Build history of the part. All positions in model axes, mm. Face numbers are marked on the shaded views. A direction names the side the tool comes from. Round coordinates to 2 decimals unless told otherwise and drop trailing zeros. Loops run counter-clockwise (first coordinate to the right, second up) from the corner with the lowest first, then second, coordinate; pieces in that order, holes last. Notation, with made-up numbers: (81.5, 10) - (90.5, 10) arc R24 cw to (90.5, 36) - close; hole circle Ø5 at (-16.5, 8). An arc over 180 degrees is marked (long way). Answer as CSV lines item,"result". Start each with the question number.
```python
from build123d import *

# Parameters (mm, degrees)
SKETCH1_W           = 54.800000096
SKETCH1_H           = 50.990000096
BOSS_EXTRUDE2_DEPTH = 2
SKETCH2_R           = 2
SKETCH2_R_2         = 1
BOSS_EXTRUDE3_DEPTH = 3
SKETCH3_W           = 54.800000096
SKETCH3_H           = 50.990000096
SKETCH3_W_2         = 50.800000096
SKETCH3_H_2         = 46.990000096
BOSS_EXTRUDE5_DEPTH = 47.45


with BuildPart() as part:
    # Sketch1 → Boss-Extrude2 (new body)
    with BuildSketch(Plane(origin=(0, 0, 0), x_dir=(1, 0, 0), z_dir=(0, 1, 0))):
        Rectangle(SKETCH1_W, SKETCH1_H)
    extrude(amount=BOSS_EXTRUDE2_DEPTH)

    # Sketch2 → Boss-Extrude3 (add)
    # profile 1 of 4: a face of its own
    with BuildSketch(Plane(origin=(0, 2, 0), x_dir=(1, 0, 0), z_dir=(0, 1, 0))):
        with Locations(Location((-22.86, 20.955, 0), (0, 0, 90))):
            Circle(SKETCH2_R)
        with Locations(Location((-22.86, 20.955, 0), (0, 0, 270))):
            Circle(SKETCH2_R_2, mode=Mode.SUBTRACT)
    # profile 2 of 4: a face of its own
    with BuildSketch(Plane(origin=(0, 2, 0), x_dir=(1, 0, 0), z_dir=(0, 1, 0))):
        with Locations(Location((22.86, 20.955, 0), (0, 0, 90))):
            Circle(SKETCH2_R)
        with Locations(Location((22.86, 20.955, 0), (0, 0, 270))):
            Circle(SKETCH2_R_2, mode=Mode.SUBTRACT)
    # profile 3 of 4: a face of its own
    with BuildSketch(Plane(origin=(0, 2, 0), x_dir=(1, 0, 0), z_dir=(0, 1, 0))):
        with Locations(Location((22.86, -20.955, 0), (0, 0, 90))):
            Circle(SKETCH2_R)
        with Locations(Location((22.86, -20.955, 0), (0, 0, 270))):
            Circle(SKETCH2_R_2, mode=Mode.SUBTRACT)
    # profile 4 of 4: a face of its own
    with BuildSketch(Plane(origin=(0, 2, 0), x_dir=(1, 0, 0), z_dir=(0, 1, 0))):
        with Locations(Location((-22.86, -20.955, 0), (0, 0, 90))):
            Circle(SKETCH2_R)
        with Locations(Location((-22.86, -20.955, 0), (0, 0, 270))):
            Circle(SKETCH2_R_2, mode=Mode.SUBTRACT)
    extrude(amount=BOSS_EXTRUDE3_DEPTH)

    # Sketch3 → Boss-Extrude5 (add)
    with BuildSketch(Plane(origin=(0, 2, 0), x_dir=(1, 0, 0), z_dir=(0, 1, 0))):
        Rectangle(SKETCH3_W, SKETCH3_H)
        Rectangle(SKETCH3_W_2, SKETCH3_H_2, mode=Mode.SUBTRACT)
    extrude(amount=BOSS_EXTRUDE5_DEPTH)


solid = part.part
```
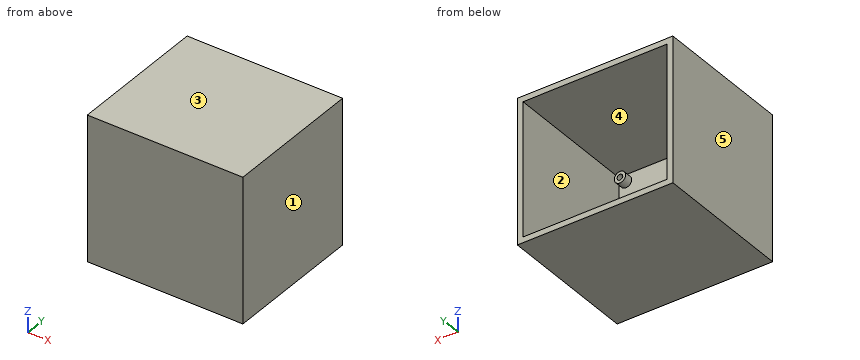
Q1. Band-saw the part on D-D, the plane z = 0.5. List the corners of the cut face in (x, y), then the cut area to 3 significant figures.
Q2. Band-saw the part on A-A, the plane y = 3.5. Give the number of separate pieces and of enclosed holes in the cut face, then the cut area to 3 significant figures.
Q3. Pin check, flat tips, straight feed: pin 1 Ø1.6 at (x, z) = (22.86, -20.955) entering from +Y; pin 2 Ø1 at (x, z) = (-13.5, 11.5) entering from -Y; pin 3 Ø1.2 at (x, z) = (24, -20.5) entering from +Y. Stop position of each tip, or through.
Q4. Band-saw the part on B-B, the plane y = 30. List the corners of the cut face in (x, z) (3 decimals), then the cut area to 3 significant figures.
Q5. Tool access for the marked faces 4 and 5: list every direction of +Z, -Z, +X, -X, +Y, -Y with a clear straight run to the whole face (end or side of a thin tool).
Q6. Wall check: probe 1 along X at (y, z) = (5.5, 7); probe 2 along Z at (x, y) = (-17, 16.5) (3 decimals); probe 3 along Z at (x, y) = (22, 4) (3 decimals). Give the ranges that are in metal, low to high. Write a range as [from, to].
Q7. Two-plate mould, pull along X, no slides. Class the marked faces 1, 2 and 3: released by +X, released by -X, zero draft, split by the parting line, or undercut.
Q8. Band-saw the part on C-C, the plane x = 10.5. List the corners of the cut face in (y, z) (3 decimals), then the cut area to 3 significant figures.
Reported:
1,outline,"(-27.4, 0) - (27.4, 0) - (27.4, 49.45) - (25.4, 49.45) - (25.4, 2) - (-25.4, 2) - (-25.4, 49.45) - (-27.4, 49.45) - close"
1,area,"299 mm2"
2,separate pieces,"5"
2,enclosed holes,"5"
2,area,"445 mm2"
3,pin 1,"stops at y = 2"
3,pin 2,"stops at y = 0"
3,pin 3,"stops at y = 5"
4,outline,"(-27.4, -25.495) - (27.4, -25.495) - (27.4, 25.495) - (-27.4, 25.495) - close; hole (-25.4, -23.495) - (25.4, -23.495) - (25.4, 23.495) - (-25.4, 23.495) - close"
4,area,"407 mm2"
5,face 4,"+Y"
5,face 5,"+Z, -Z, -X, +Y, -Y"
6,probe 1,"x = [-27.4, -25.4], [25.4, 27.4]"
6,probe 2,"z = [-25.495, -23.495], [23.495, 25.495]"
6,probe 3,"z = [-25.495, -23.495], [-22.761, -21.465], [-20.445, -19.149], [19.149, 20.445], [21.465, 22.761], [23.495, 25.495]"
7,face 1,"released by +X"
7,face 2,"undercut"
7,face 3,"zero draft"
8,outline,"(0, -25.495) - (49.45, -25.495) - (49.45, -23.495) - (2, -23.495) - (2, 23.495) - (49.45, 23.495) - (49.45, 25.495) - (0, 25.495) - close"
8,area,"292 mm2"
